Drawing for the job (mm, zero at the part's lowest x, y, z). A direction names the side the tool comes from. Give positions to 0.01 mm unless a question says otherwise; leave off trailing zeros. Order: outer loops, then holes, each group sorted by start corner. A loop starts at its lowest first (then second) coordinate and runs counter-clockwise, first axis right, second up. Notation, with made-up numbers: (39, 8) -> (71, 8) arc R20 ccw to (71, 41) -> close; hole circle Ø1 at (6, -3.75). An arc over 180 degrees is marked (long way). Use one line per item in the form item = value. Start each with the question number.
1) Mould opens along X. For the marked faces 1, 2 and 3 say: pulls with the +X half, pulls with the -X half, needs draft (parallel to the pull), parting line crosses it, or undercut.
2) Drop flat-ended pins along their axis: P1, Ø8.5, axis at x = 98.5, z = 22, coming from the -Y side; P2, Ø5, axis at x = 97.5, z = 28, coming from the +Y side; P3, Ø8, axis at y = 13, z = 27, coming from the +X side. Give the stop position or say it passes through.
3) Probe line 1 (Z direction, x = 95, y = 18.75); line 2 (Z direction, x = 56, y = 31); line 3 (Y direction, x = 27.5, z = 26). List the from-to ranges inside material, lowest first.
4) Cut at A-A, the plane y = 20. Give the cut face in (x, z).
5) Cut at D-D, the plane y = 29.5. Give the cut face in (x, z).
6) Cut at C-C, the plane y = 6.5. Give the cut face in (x, z).
7) Cut at B-B, the plane x = 17. Give the cut face in (y, z), and give its area (3 significant figures).
8) Tool access for the marked faces 4, 5 and 6: list every direction of +Z, -Z, +X, -X, +Y, -Y with a clear straight run to the whole face (end or side of a thin tool).
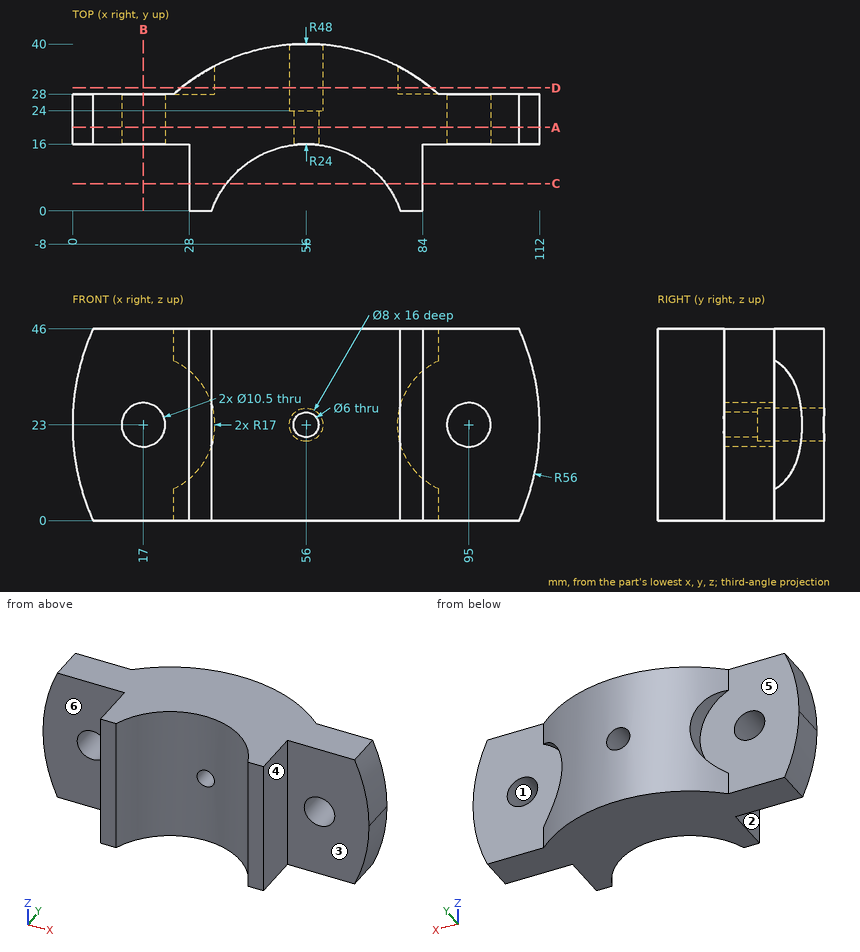
Result:
q1.face_1 = undercut
q1.face_2 = pulls with the -X half
q1.face_3 = needs draft
q2.P1 = 16
q2.P2 = 28
q2.P3 = 111.98
q3.line_1 = 0 to 17.75, 28.25 to 46
q3.line_2 = 0 to 19, 27 to 46
q3.line_3 = 16 to 28
q4.outline = (4.94, 0) -> (107.06, 0) arc R56 ccw to (107.06, 46) -> (4.94, 46) arc R56 ccw to start; hole circle Ø10.5 at (17, 23); hole circle Ø6 at (56, 23); hole circle Ø10.5 at (95, 23)
q5.outline = (26.04, 0) -> (85.96, 0) -> (85.96, 8.6) arc R17 cw to (85.96, 37.4) -> (85.96, 46) -> (26.04, 46) -> (26.04, 37.4) arc R17 cw to (26.04, 8.6) -> close; hole circle Ø8 at (56, 23)
q6.outline = (28, 0) -> (36.88, 0) -> (36.88, 46) -> (28, 46) -> close; (75.12, 0) -> (84, 0) -> (84, 46) -> (75.12, 46) -> close
q7.outline = (16, 0) -> (28, 0) -> (28, 17.75) -> (16, 17.75) -> close; (16, 28.25) -> (28, 28.25) -> (28, 46) -> (16, 46) -> close
q7.area = 426 mm²
q8.face_4 = +Z, -Z, +X, -Y
q8.face_5 = -X, +Y
q8.face_6 = +Z, -Z, -X, -Y
